Work out the finished part from the listing and answer in its coordinate system (mm). Face numbers are marked on the shaded views. A direction names the side the tool comes from. Coordinates: 2 decimals unless noted, no trailing zeros. Loops run counter-clockwise (first coordinate to the right, second up) from the corner with the lowest first, then second, coordinate; pieces in that order, holes last. Notation, with made-up numbers: (19.25, 77.25) -> (41.25, 77.25) arc R16 cw to (41.25, 84.25) -> close; hole circle Ø7 at (1.25, -4). An arc over 180 degrees is marked (long way). Use a Markdown table: item, result.
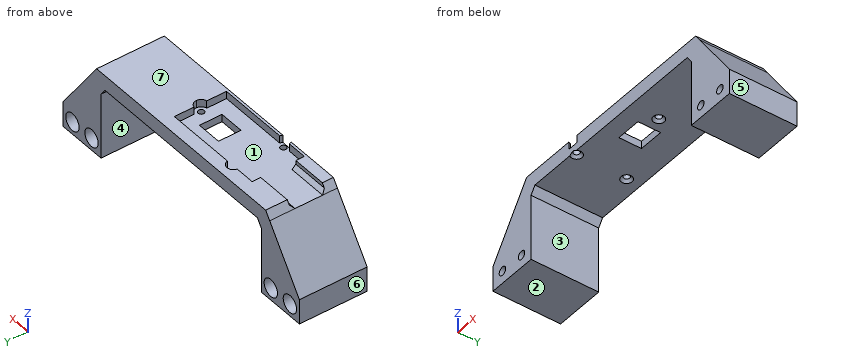
from build123d import *
from OCP.BRepFilletAPI import BRepFilletAPI_MakeChamfer

# Parameters (mm, degrees)
BOSS_EXTRUDE1_DEPTH                                 = 27
SKETCH2_W                                           = 10
SKETCH2_H                                           = 9
CUT_EXTRUDE1_DEPTH                                  = 75.920374398
CBORE_FOR_M3_PAN_HEAD_SCREW1_D                      = 3.4
CBORE_FOR_M3_PAN_HEAD_SCREW1_CBORE_D                = 7
CBORE_FOR_M3_PAN_HEAD_SCREW1_CBORE_DEPTH            = 8
CSK_FOR_M2_COUNTERSUNK_FLAT_HEAD_SCREW1_D           = 2.4
CSK_FOR_M2_COUNTERSUNK_FLAT_HEAD_SCREW1_CSINK_D     = 4.4
CSK_FOR_M2_COUNTERSUNK_FLAT_HEAD_SCREW1_CSINK_ANGLE = 90
BOSS_EXTRUDE2_DEPTH                                 = 3
CHAMFER1_SIZE                                       = 1.5
CHAMFER2_SIZE                                       = 3
CHAMFER2_SIZE_2                                     = 2.100622615


with BuildPart() as part:
    # Sketch1 → Boss-Extrude1 (new body)
    with BuildSketch(Plane(origin=(0, 0, 0), x_dir=(1, 0, 0), z_dir=(0, 1, 0))):
        Polygon((39.975582768, 0), (0, 0), (0, -3), (46.420382275, -3), (62, 19.25), (62, 29.25), (42, 29.25), (42, 2.891167435), align=None)
        Polygon((0, -3), (0, 0), (-39.975582768, 0), (-42, 2.891167435), (-42, 29.25), (-62, 29.25), (-62, 19.25), (-46.420382275, -3), align=None)
    extrude(amount=BOSS_EXTRUDE1_DEPTH)

    # Sketch2 → Cut-Extrude1 (cut, through all)
    with BuildSketch(Plane.XY.offset(3)):
        with Locations((0, 11.4)):
            Rectangle(SKETCH2_W, SKETCH2_H)
    extrude(amount=-CUT_EXTRUDE1_DEPTH, mode=Mode.SUBTRACT)

    # CBORE for M3 Pan Head Screw1 (through all)
    with Locations(Plane(origin=(0, 27, 0), x_dir=(1, 0, 0), z_dir=(0, 1, 0))):
        with Locations((-57, 24.25), (-47, 24.25), (47, 24.25), (57, 24.25)):
            CounterBoreHole(CBORE_FOR_M3_PAN_HEAD_SCREW1_D / 2, CBORE_FOR_M3_PAN_HEAD_SCREW1_CBORE_D / 2, CBORE_FOR_M3_PAN_HEAD_SCREW1_CBORE_DEPTH)

    # CSK for M2 Countersunk Flat Head Screw1 (through all)
    with Locations(Plane(origin=(0, 0, 0), x_dir=(1, 0, 0), z_dir=(0, 0, -1))):
        with Locations((-20, -21.400004303), (-20, -1.4), (10, -11.4)):
            CounterSinkHole(CSK_FOR_M2_COUNTERSUNK_FLAT_HEAD_SCREW1_D / 2, CSK_FOR_M2_COUNTERSUNK_FLAT_HEAD_SCREW1_CSINK_D / 2, counter_sink_angle=CSK_FOR_M2_COUNTERSUNK_FLAT_HEAD_SCREW1_CSINK_ANGLE)

    # Sketch7 → Boss-Extrude2 (add)
    with BuildSketch(Plane.XY.offset(3)):
        with BuildLine():
            Line((-30.4, 18.4), (-30.4, 21.8))
            Line((-30.4, 21.8), (-22.518432735, 21.8))
            ThreePointArc((-22.518432735, 21.8), (-20, 23.950004303), (-17.481567265, 21.8))
            Line((-17.481567265, 21.8), (10.4, 21.8))
            Line((10.4, 21.8), (10.4, 13.918432052))
            ThreePointArc((10.4, 13.918432052), (11.939394235, 13.055672069), (12.55, 11.4))
            ThreePointArc((12.55, 11.4), (11.939394235, 9.744327931), (10.4, 8.881567948))
            Line((10.4, 8.881567948), (10.4, 1))
            Line((10.4, 1), (-17.481567948, 1))
            ThreePointArc((-17.481567948, 1), (-17.621968265, 0.479421341), (-17.868685851, 0))
            Line((-17.868685851, 0), (46.420382275, 0))
            Line((46.420382275, 0), (46.420382275, 27))
            Line((46.420382275, 27), (-46.420382275, 27))
            Line((-46.420382275, 27), (-46.420382275, 18.4))
            Line((-46.420382275, 18.4), (-30.4, 18.4))
        make_face()
        with BuildLine():
            Line((-30.4, 1), (-30.4, 4.4))
            Line((-30.4, 4.4), (-46.420382275, 4.4))
            Line((-46.420382275, 4.4), (-46.420382275, 0))
            Line((-46.420382275, 0), (-22.131314149, 0))
            ThreePointArc((-22.131314149, 0), (-22.378031735, 0.479421341), (-22.518432052, 1))
            Line((-22.518432052, 1), (-30.4, 1))
        make_face()
    extrude(amount=BOSS_EXTRUDE2_DEPTH)

    # Chamfer1
    chamfer1_edges = [part.edges().sort_by_distance(p)[0] for p in [
        (-38.410191137, 18.4, 3),
        (-38.410191137, 4.4, 3),
    ]]
    chamfer(chamfer1_edges, length=CHAMFER1_SIZE)

    # Chamfer2
    chamfer2_edges_1 = [part.edges().sort_by_distance(p)[0] for p in [
        (46.420382275, 13.5, 6),
    ]]
    chamfer2_side_1 = [part.faces().sort_by_distance(p)[0] for p in [
        (46.420382275, 13.5, 5.957987548),
    ]]
    chamfer2_edges_2 = [part.edges().sort_by_distance(p)[0] for p in [
        (-46.420382275, 22.7, 6),
    ]]
    chamfer2_side_2 = [part.faces().sort_by_distance(p)[0] for p in [
        (-46.378369823, 22.7, 6),
    ]]
    chamfer2_edges_3 = [part.edges().sort_by_distance(p)[0] for p in [
        (-46.420382275, 2.2, 6),
    ]]
    chamfer2_side_3 = [part.faces().sort_by_distance(p)[0] for p in [
        (-46.378369823, 2.2, 6),
    ]]
    chamfer2 = BRepFilletAPI_MakeChamfer(part.part.solid().wrapped)
    for e in chamfer2_edges_1:
        chamfer2.Add(CHAMFER2_SIZE - 0.0001, CHAMFER2_SIZE_2 - 0.0001, e.wrapped, chamfer2_side_1[0].wrapped)
    for e in chamfer2_edges_2:
        chamfer2.Add(CHAMFER2_SIZE_2 - 0.0001, CHAMFER2_SIZE - 0.0001, e.wrapped, chamfer2_side_2[0].wrapped)
    for e in chamfer2_edges_3:
        chamfer2.Add(CHAMFER2_SIZE_2 - 0.0001, CHAMFER2_SIZE - 0.0001, e.wrapped, chamfer2_side_3[0].wrapped)
    add(Compound.cast(chamfer2.Shape()), mode=Mode.REPLACE)  # a hair under: the kernel refuses the full size


solid = part.part
Q1. Section A-A on y = 25.25 is taken. State how many separate pieces and enclosed holes the cut face has, and give its area (3 significant figures).
Solved:
| item | result |
|---|---|
| separate pieces | 1 |
| enclosed holes | 4 |
| area | 1,320 mm² |
Q2. Section D-D on x = 57 is taken. Determine the outline of the cut face in (y, z), and give its area (3 significant figures).
Solved:
| item | result |
|---|---|
| outline | (0, -29.25) -> (27, -29.25) -> (27, -27.75) -> (19, -27.75) -> (19, -25.95) -> (0, -25.95) -> close; (0, -22.55) -> (19, -22.55) -> (19, -20.75) -> (27, -20.75) -> (27, -12.11) -> (0, -12.11) -> close |
| area | 342 mm² |
Q3. Consider line 1 (X direction, y = 13, z = -24.25); line 2 (X direction, y = 23.25, z = -24.25); line 3 (X direction, y = 13.75, z = -27.5). Determine where each line is inside the solid, lowest interval first. Write a range as [from, to].
Solved:
| item | result |
|---|---|
| line 1 | [-62, -58.7], [-55.3, -48.7], [-45.3, -42], [42, 45.3], [48.7, 55.3], [58.7, 62] |
| line 2 | [-62, -60.5], [-53.5, -50.5], [-43.5, -42], [42, 43.5], [50.5, 53.5], [60.5, 62] |
| line 3 | [-62, -42], [42, 62] |
Q4. Determine the mould class of the marked faces 4, 5, 6 and 7 for opening direction X: pulls with the +X half, pulls with the -X half, needs draft (parallel to the pull), parting line crosses it, or undercut.
Solved:
| item | result |
|---|---|
| face 4 | undercut |
| face 5 | pulls with the +X half |
| face 6 | pulls with the -X half |
| face 7 | needs draft |
Q5. Given pin 1 Ø2 at (x, y) = (-28, 6.5) entering from -Z; pin 2 Ø1.5 at (y, z) = (22.5, 2) entering from +X; pin 3 Ø1.5 at (y, z) = (19.5, 4.5) entering from +X; pin 4 Ø2 at (x, z) = (-47, -24.25) entering from -Y, each flat-ended and moving along its own axis, determine where each tip first touches the part or whether it passes through.
Solved:
| item | result |
|---|---|
| pin 1 | z = 0 |
| pin 2 | x = 47.65 |
| pin 3 | x = 45.9 |
| pin 4 | through |
Q6. Section B-B on x = -25 is taken. Determine the outline of the cut face in (y, z), and give its area (3 significant figures).
Solved:
| item | result |
|---|---|
| outline | (0, 0) -> (27, 0) -> (27, 6) -> (21.8, 6) -> (21.8, 3) -> (1, 3) -> (1, 6) -> (0, 6) -> close |
| area | 99.6 mm² |
Q7. Section C-C on z = -14 is taken. Determine the outline of the cut face in (x, y), and give its area (3 significant figures).
Solved:
| item | result |
|---|---|
| outline | (-58.32, 0) -> (-42, 0) -> (-42, 27) -> (-58.32, 27) -> close; (42, 0) -> (58.32, 0) -> (58.32, 27) -> (42, 27) -> close |
| area | 881 mm² |
Q8. For the marked faces 1, 2 and 3, determine the directions among +Z, -Z, +X, -X, +Y, -Y from which every point of the face is accessible in a straight line to the end or side of a thin tool.
Solved:
| item | result |
|---|---|
| face 1 | +Z |
| face 2 | -Z, +X, -X, +Y, -Y |
| face 3 | -Z, +Y, -Y |
